```python
from build123d import *

# Parameters (mm, degrees)
SKETCH1_W           = 22.5
SKETCH1_H           = 22.5
BOSS_EXTRUDE1_DEPTH = 20
SKETCH5_W           = 5
SKETCH5_H           = 4
SKETCH3_W           = 18.5
SKETCH3_H           = 18.5
CUT_EXTRUDE5_DEPTH  = 6
CUT_EXTRUDE5_TAPER  = 8
SKETCH14_W          = 16.813509984
SKETCH14_H          = 16.813509984
CUT_EXTRUDE6_DEPTH  = 2
CUT_EXTRUDE7_REACH  = 14
SKETCH15_W          = 14.313509984
SKETCH15_H          = 14.313509984


with BuildPart() as part:
    # Sketch1 → Boss-Extrude1 (new body)
    with BuildSketch(Plane(origin=(0, 0, 0), x_dir=(1, 0, 0), z_dir=(0, 1, 0))):
        Rectangle(SKETCH1_W, SKETCH1_H)
    extrude(amount=BOSS_EXTRUDE1_DEPTH)

    # Sweep1: sweep along a path in Sketch6
    with BuildLine(Plane(origin=(0, 0, 0), x_dir=(0, 0, -1), z_dir=(1, 0, 0))) as sweep1_path:
        Line((11.25, 16), (14.25, 16))
        ThreePointArc((14.25, 16), (16.546100594, 16.456722805), (18.492640687, 17.757359313))
    # Sketch5 → Sweep1 (sweep)
    with BuildSketch(Plane(origin=(0, 0, -11.25), x_dir=(-1, 0, 0), z_dir=(0, 0, -1))):
        with Locations((0, 16)):
            Rectangle(SKETCH5_W, SKETCH5_H)
    sweep1 = sweep(path=sweep1_path.line)

    # Mirror1: Sweep1 across plane
    add(sweep1.mirror(Plane.XY))

    # Sketch3 → Cut-Extrude5 (cut)
    with BuildSketch(Plane.XZ):
        Rectangle(SKETCH3_W, SKETCH3_H)
    extrude(amount=-CUT_EXTRUDE5_DEPTH, taper=CUT_EXTRUDE5_TAPER, mode=Mode.SUBTRACT)

    # Sketch14 → Cut-Extrude6 (cut)
    with BuildSketch(Plane.XZ.offset(-6)):
        Rectangle(SKETCH14_W, SKETCH14_H)
    extrude(amount=-CUT_EXTRUDE6_DEPTH, mode=Mode.SUBTRACT)

    # Sketch15 → Cut-Extrude7 (cut, up to next)
    with BuildSketch(Plane.XZ.offset(-8), mode=Mode.PRIVATE) as cut_extrude7_sk1:
        Rectangle(SKETCH15_W, SKETCH15_H)
    cut_extrude7_tool1 = extrude(cut_extrude7_sk1.sketch, amount=-CUT_EXTRUDE7_REACH, mode=Mode.PRIVATE) & part.part
    add(cut_extrude7_tool1.solids().sort_by_distance((0, 8, 0))[0], mode=Mode.SUBTRACT)


solid = part.part
```
The model under review builds one solid part; all positions refer to its coordinate system, in mm. A direction names the side the tool comes from. Coordinates: 2 decimals unless noted, no trailing zeros. Order: outer loops, then holes, each group sorted by start corner. A loop starts at its lowest first (then second) coordinate and runs counter-clockwise, first axis right, second up. Notation, with made-up numbers: M 39.25,-22.75 L 88.25,-22.75 A13 ccw 88.25,-10.75 Z; hole C 81.5,10 d2. An arc over 180 degrees is marked long. One line per question, with ' | ' between items.
(1) Insertion check: pin 1 (2.5 mm diameter, centred on y = 15.5, z = -14, fed in from +X); pin 2 (2.5 mm diameter, centred on x = 0, z = 13.5, fed in from -Y); pin 3 (3.5 mm diameter, centred on x = -2, y = 13, fed in from +Z). Each pin has a flat end and moves straight along its axis. Give the tip position at first contact, or say it passes through.
Geometry results:
pin 1: stops at x = 2.5 | pin 2: stops at y = 14 | pin 3: stops at z = 17.63
(2) Machinability: for faces 1 (the face through (7.157, 14, 0)), 2 (the face through (7.4, 8, 0.1)), 3 (the face through (2.5, 16, 15)), 4 (the face through (0.035, 18.296, 15.76)), which of the approach directions +Z, -Z, +X, -X, +Y, -Y give a long, thin tool a straight path to every point of the face, cutting with its end or side? Answer none if there is none.
Geometry results:
face 1: +Y, -Y | face 2: -Y | face 3: +Z, +X, +Y, -Y | face 4: +X, -X, +Y
(3) For probe 1 along Z at (x, y) = (0.75, 6.5); probe 2 along Z at (x, y) = (3.5, 18), list the stretches that pass through material, from the lowest coordinate up. Write a range as from..to.
Geometry results:
probe 1: z = -11.25..-8.41, 8.41..11.25 | probe 2: z = -11.25..-7.16, 7.16..11.25
(4) Add section A-A, the plane y = 9.5. Write out the cut boundary in (x, z), then the cut area to 3 significant figures.
Geometry results:
outline: M -11.25,-11.25 L 11.25,-11.25 L 11.25,11.25 L -11.25,11.25 Z; hole M -7.16,-7.16 L 7.16,-7.16 L 7.16,7.16 L -7.16,7.16 Z | area: 301 mm²
(5) The part is to be moulded in two halves that separate along X. For faces 5 (the face through (0, 7, -8.407)), 6 (the face through (0, 20, -8)), 7 (the face through (-11.25, 10, 0)), say which applies: +X half, -X half, draft (parallel to the pull), parting line (faces both ways), or undercut.
Geometry results:
face 5: undercut | face 6: draft | face 7: -X half
(6) Add section B-B, the plane z = -12.5. Write out the cut boundary in (x, y).
Geometry results:
outline: M -2.5,14 L 2.5,14 L 2.5,18 L -2.5,18 Z
(7) Add section C-C, the plane y = 15.25. Write out the cut boundary in (x, z), then the cut area to 3 significant figures.
Geometry results:
outline: M -11.25,-11.25 L -2.5,-11.25 L -2.5,-18.54 L 2.5,-18.54 L 2.5,-11.25 L 11.25,-11.25 L 11.25,11.25 L 2.5,11.25 L 2.5,18.54 L -2.5,18.54 L -2.5,11.25 L -11.25,11.25 Z; hole M -7.16,-7.16 L 7.16,-7.16 L 7.16,7.16 L -7.16,7.16 Z | area: 374 mm²
